CAD build for the part. Positions are in the model's coordinates, mm. Face numbers are marked on the shaded views. Round coordinates to 2 decimals unless told otherwise and drop trailing zeros. Order: outer loops, then holes, each group sorted by start corner. A loop starts at its lowest first (then second) coordinate and runs counter-clockwise, first axis right, second up. Notation, with made-up numbers: M 27.5,-32.75 L 51.5,-32.75 A16 ccw 51.5,-1.75 Z; hole C 51,56 d11. An arc over 180 degrees is marked long. Answer as a JSON object with one key per item and string values.
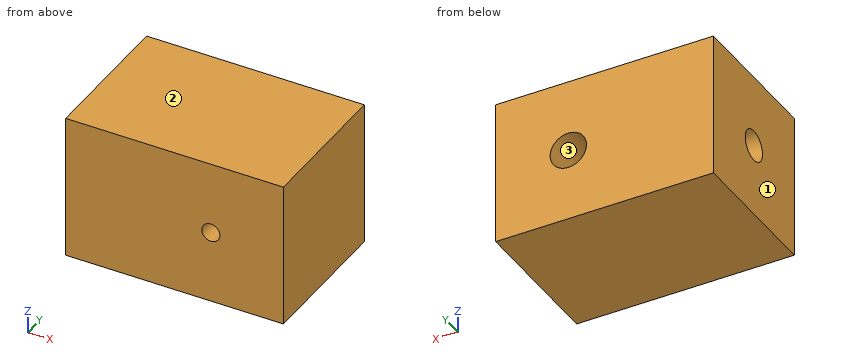
```python
from build123d import *

# Parameters (mm, degrees)
SKETCH1_W                   = 38.1
SKETCH1_H                   = 25.4
BOSS_EXTRUDE1_DEPTH         = 25.4
SKETCH3_R                   = 1.5875
CUT_EXTRUDE2_DEPTH          = 25.4
F_1_4_28_TAPPED_HOLE1_D     = 5.4102
F_1_4_28_TAPPED_HOLE1_DEPTH = 17.23
F_1_4_28_TAPPED_HOLE1_TIP   = 1.625388061
SKETCH2_R                   = 3.18
CUT_EXTRUDE6_DEPTH          = 15.875
SKETCH8_R                   = 1.5875
CUT_EXTRUDE7_DEPTH          = 35.1957966


with BuildPart() as part:
    # Sketch1 → Boss-Extrude1 (new body)
    with BuildSketch(Plane(origin=(0, 0, 0), x_dir=(1, 0, 0), z_dir=(0, 1, 0))):
        Rectangle(SKETCH1_W, SKETCH1_H)
    extrude(amount=BOSS_EXTRUDE1_DEPTH)

    # Sketch3 → Cut-Extrude2 (cut)
    with BuildSketch(Plane.ZY.offset(19.05)):
        with Locations((0, 12.7)):
            Circle(SKETCH3_R)
    extrude(amount=-CUT_EXTRUDE2_DEPTH, mode=Mode.SUBTRACT)

    # 1/4-28 Tapped Hole1
    with Locations(Plane.ZY.offset(19.05)):
        with Locations((0, 12.7)):
            Hole(F_1_4_28_TAPPED_HOLE1_D / 2, depth=F_1_4_28_TAPPED_HOLE1_DEPTH)
            with Locations((0, 0, -(F_1_4_28_TAPPED_HOLE1_DEPTH + F_1_4_28_TAPPED_HOLE1_TIP / 2))):  # 118° drill point
                Cone(0, F_1_4_28_TAPPED_HOLE1_D / 2, F_1_4_28_TAPPED_HOLE1_TIP, mode=Mode.SUBTRACT)

    # Sketch2 → Cut-Extrude6 (cut)
    with BuildSketch(Plane(origin=(0, 25.4, 0), x_dir=(1, 0, 0), z_dir=(0, 1, 0))):
        with Locations(Location((6.35, 0, 0), (0, 0, 270))):
            Circle(SKETCH2_R)
    extrude(amount=-CUT_EXTRUDE6_DEPTH, mode=Mode.SUBTRACT)

    # Sketch8 → Cut-Extrude7 (cut, through all)
    with BuildSketch(Plane.XZ):
        with Locations(Location((6.35, 0, 0), (0, 0, 270))):
            Circle(SKETCH8_R)
    extrude(amount=-CUT_EXTRUDE7_DEPTH, mode=Mode.SUBTRACT)


solid = part.part
```
Item 1: Wall check: line 1 along X through (y, z) = (3, 0); line 2 along Z through (x, y) = (6.5, 21); line 3 along X through (y, z) = (19, 0). Give the ranges that are in metal, low to high. Write a range as [from, to].
Worked answers:
{"line 1": "x = [-19.05, 4.76], [7.94, 19.05]", "line 2": "z = [-12.7, -3.18], [3.18, 12.7]", "line 3": "x = [-19.05, 3.17], [9.53, 19.05]"}
Item 2: Saw through at C-C on x = 6.35. List the corners of the cut face in (y, z) (1 decimal), and give its area (3 significant figures).
Worked answers:
{"outline": "M 0,-12.7 L 25.4,-12.7 L 25.4,-3.2 L 9.5,-3.2 L 9.5,-1.6 L 0,-1.6 Z; M 0,1.6 L 9.5,1.6 L 9.5,3.2 L 25.4,3.2 L 25.4,12.7 L 0,12.7 Z", "area": "514 mm2"}
Item 3: Two-plate mould, pull along X, no slides. Class the marked faces 1, 2 and 3: released by +X, released by -X, zero draft, split by the parting line, or undercut.
Worked answers:
{"face 1": "released by -X", "face 2": "zero draft", "face 3": "undercut"}
Item 4: Drop a flat-ended pin along its axis: pin 1 Ø3.5 at (x, z) = (6.35, 0) entering from +Y (3 decimals). Give the stop position or say it passes through.
Worked answers:
{"pin 1": "stops at y = 9.525"}
Item 5: Saw through at B-B on y = 21. List the corners of the cut face in (x, z).
Worked answers:
{"outline": "M -19.05,-12.7 L 19.05,-12.7 L 19.05,12.7 L -19.05,12.7 Z; hole C 6.35,0 d6.36"}
Item 6: Saw through at D-D on y = 12.7. List the corners of the cut face in (x, z), and give its area (3 significant figures).
Worked answers:
{"outline": "M -19.05,-12.7 L 19.05,-12.7 L 19.05,12.7 L -19.05,12.7 L -19.05,2.71 L -1.82,2.71 L -1.15,1.59 L 3.59,1.59 A3.18 cw long 3.59,-1.59 L -1.15,-1.59 L -1.82,-2.71 L -19.05,-2.71 Z", "area": "826 mm2"}
Item 7: Saw through at A-A on z = 0. State how many separate pieces and enclosed holes the cut face has, and give its area (3 significant figures).
Worked answers:
{"separate pieces": "3", "enclosed holes": "0", "area": "727 mm2"}
